Work out the finished part from the listing and answer in its coordinate system (mm). A direction names the side the tool comes from. Give positions to 0.01 mm unless a question says otherwise; leave off trailing zeros. Loops run counter-clockwise (first coordinate to the right, second up) from the corner with the lowest first, then second, coordinate; pieces in that order, holes last. Notation, with made-up numbers: (18, -3.5) - (65, -3.5) arc R19 ccw to (65, 18.5) - close; hole circle Ø6 at (24.25, 46). An arc over 180 degrees is marked (long way). Use CSV: the item, a comma, the result in double quotes.
from build123d import *

# Parameters (mm, degrees)
BOSS_EXTRUDE1_DEPTH = 8.001
CUT_EXTRUDE1_DEPTH  = 7.6962
CUT_EXTRUDE2_DEPTH  = 7.6962
SKETCH8_W           = 32.004
SKETCH8_H           = 15.3924
CUT_EXTRUDE3_DEPTH  = 7.6962
BOSS_EXTRUDE2_DEPTH = 3.0734


with BuildPart() as part:
    # Sketch1 → Boss-Extrude1 (new body, symmetric)
    with BuildSketch(Plane(origin=(0, 0, 0), x_dir=(0, 0, -1), z_dir=(1, 0, 0))):
        Polygon((-3.8481, 4.34848), (-3.8481, 0), (3.8481, 0), (3.8481, 4.34848), (3.6195, 3.99288), (3.1115, 4.50088), (2.6035, 3.99288), (2.0955, 4.50088), (1.5875, 3.99288), (1.0795, 4.50088), (0.5715, 3.99288), (0.0635, 4.50088), (-0.4445, 3.99288), (-0.9525, 4.50088), (-1.4605, 3.99288), (-1.9685, 4.50088), (-2.4765, 3.99288), (-2.9845, 4.50088), (-3.4925, 3.99288), align=None)
    extrude(amount=BOSS_EXTRUDE1_DEPTH, both=True)

    # Sketch2 → Cut-Extrude1 (cut, symmetric)
    with BuildSketch(Plane.XY):
        Polygon((-10.541, 2.99974), (-10.541, -2.99974), (0, -2.99974), (0, 0), (-5.00126, 0), (-8.001, 2.99974), align=None)
    extrude(amount=CUT_EXTRUDE1_DEPTH, both=True, mode=Mode.SUBTRACT)

    # Sketch5 → Cut-Extrude2 (cut, symmetric)
    with BuildSketch(Plane.XY):
        Polygon((0, 0), (0, -2.99974), (10.541, -2.99974), (10.541, 2.99974), (8.001, 2.99974), (5.00126, 0), align=None)
    extrude(amount=CUT_EXTRUDE2_DEPTH, both=True, mode=Mode.SUBTRACT)

    # Sketch8 → Cut-Extrude3 (cut)
    with BuildSketch(Plane(origin=(0, 0, 0), x_dir=(1, 0, 0), z_dir=(0, 1, 0))):
        Rectangle(SKETCH8_W, SKETCH8_H)
        with BuildLine():
            Line((-6.985, -3.8481), (6.385094721, -3.8481))
            ThreePointArc((6.385094721, -3.8481), (6.939045596, -3.683800903), (7.313835784, -3.244041788))
            ThreePointArc((7.313835784, -3.244041788), (7.827323972, -1.658010991), (8.001, 0))
            Line((8.001, 0), (8.001, 2.8321))
            ThreePointArc((8.001, 2.8321), (7.70342049, 3.55052049), (6.985, 3.8481))
            Line((6.985, 3.8481), (-6.385094721, 3.8481))
            ThreePointArc((-6.385094721, 3.8481), (-6.939045596, 3.683800903), (-7.313835784, 3.244041788))
            ThreePointArc((-7.313835784, 3.244041788), (-7.827323972, 1.658010991), (-8.001, 0))
            Line((-8.001, 0), (-8.001, -2.8321))
            ThreePointArc((-8.001, -2.8321), (-7.70342049, -3.55052049), (-6.985, -3.8481))
        make_face(mode=Mode.SUBTRACT)
    extrude(amount=CUT_EXTRUDE3_DEPTH, mode=Mode.SUBTRACT)

    # Sketch9 → Boss-Extrude2 (add)
    with BuildSketch(Plane(origin=(0, 6.1468, 0), x_dir=(1, 0, 0), z_dir=(0, 1, 0))):
        with BuildLine():
            Line((-2.8321, -3.8481), (0, -3.8481))
            ThreePointArc((0, -3.8481), (2.721017605, -2.721017605), (3.8481, 0))
            Line((3.8481, 0), (3.8481, 2.8321))
            ThreePointArc((3.8481, 2.8321), (3.55052049, 3.55052049), (2.8321, 3.8481))
            Line((2.8321, 3.8481), (0, 3.8481))
            ThreePointArc((0, 3.8481), (-2.721017605, 2.721017605), (-3.8481, 0))
            Line((-3.8481, 0), (-3.8481, -2.8321))
            ThreePointArc((-3.8481, -2.8321), (-3.55052049, -3.55052049), (-2.8321, -3.8481))
        make_face()
    extrude(amount=-BOSS_EXTRUDE2_DEPTH)

    # Sketch10 → Cut-Revolve1 (revolve, cut)
    with BuildSketch(Plane(origin=(0, 6.1468, 0), x_dir=(-1, 0, 0), z_dir=(0, 0, 1))):
        Polygon((2.50000008, 6.1468), (0, 6.1468), (0, 0), (2.50000008, 0), (2.06699993, 0.433000023), (2.06699993, 5.713799977), align=None)
    revolve(axis=Axis((0, 6.45414, 0), (0, -1, 0)), mode=Mode.SUBTRACT)


solid = part.part
Item 1: A cutting plane is placed at A-A on y = 2.5. Determine the outline of the cut face in (x, z) (3 decimals).
Determined:
outline,"(-7.501, -2.783) arc R8.001 ccw to (-7.314, -3.244) arc R1.016 ccw to (-6.385, -3.848) - (6.985, -3.848) arc R1.016 ccw to (7.501, -3.707) - (7.501, 2.783) arc R8.001 ccw to (7.314, 3.244) arc R1.016 ccw to (6.385, 3.848) - (-6.985, 3.848) arc R1.016 ccw to (-7.501, 3.707) - close; hole circle Ø4.134 at (0, 0)"
Item 2: A cutting plane is placed at B-B on x = 5.25. Determine the outline of the cut face in (y, z).
Determined:
outline,"(0.25, -3.85) - (4.35, -3.85) - (3.99, -3.62) - (4.5, -3.11) - (3.99, -2.6) - (4.5, -2.1) - (3.99, -1.59) - (4.5, -1.08) - (3.99, -0.57) - (4.5, -0.06) - (3.99, 0.44) - (4.5, 0.95) - (3.99, 1.46) - (4.5, 1.97) - (3.99, 2.48) - (4.5, 2.98) - (3.99, 3.49) - (4.35, 3.85) - (0.25, 3.85) - close"
Item 3: Find the intervals of material crossed by line 1 (Z direction, x = 0, y = 2.55); line 2 (Z direction, x = -1.5, y = 2.5); line 3 (X direction, y = 5.5, z = -0.5), in increasing order.
Determined:
line 1,"z = -3.85 to -2.07, 2.07 to 3.85"
line 2,"z = -3.85 to -1.42, 1.42 to 3.85"
line 3,"x = -3.82 to -2.01, 2.01 to 3.85"
Item 4: For faces 4 (the flat face through (3.848, 5, -1)), 5 (the cylindrical face through (-6.93, 3.19, -3.69)), 6 (the flat face through (-3.848, 5, 1)), determine the directions among +Z, -Z, +X, -X, +Y, -Y from which every point of the face is accessible in a straight line to the end or side of a thin tool.
Determined:
face 4,"+X, +Y"
face 5,"-Z, -X, +Y, -Y"
face 6,"-X, +Y"
Item 5: Given P1, Ø1.7, axis at y = 5.5, z = 1.5, coming from the -X side; P2, Ø1.5, axis at y = 2.5, z = 1, coming from the +X side; P3, Ø1, axis at x = 6, z = -1.5, coming from the -Y side, each flat-ended and moving along its own axis, determine where each tip first touches the part or whether it passes through.
Determined:
P1,"stops at x = -3.85"
P2,"stops at x = 7.99"
P3,"stops at y = 0.5"
Item 6: The mould has two halves that part along Z. Classify faces 1 (the flat face through (-6, 1, 0)), 2 (the cylindrical face through (7.711, 3.504, -3.543)), 3 (the cylindrical face through (0.448, 3.036, 2.018)): pulls with the +Z half, pulls with the -Z half, needs draft (parallel to the pull), parting line crosses it, or undercut.
Determined:
face 1,"needs draft"
face 2,"pulls with the -Z half"
face 3,"undercut"
